Autodesk Inventor part; units mm, degrees
ref_plane "YZ Plane" through (0, 0, 0) normal (1, 0, 0) x (0, 1, 0)
ref_plane "XZ Plane" through (0, 0, 0) normal (0, 1, 0) x (-1, 0, 0)
ref_plane "XY Plane" through (0, 0, 0) normal (0, 0, 1) x (1, 0, 0)
sketch "Sketch1" plane through (0, 0, 0) normal (0, 1, 0) x (-1, 0, 0)
  line L0 (13, -39.6468) -> (13, 41.6738)
  line L1 (13, 41.6738) -> (-0.1234, 53.6991)
  line L2 (-0.1234, 53.6991) -> (-13, 39.6468)
  line L3 (-13, 39.6468) -> (-13, -41.6738)
  line L4 (-13, -41.6738) -> (0.1234, -53.6991)
  line L5 (0.1234, -53.6991) -> (13, -39.6468)
  line L6 (-9.6864, 40.3026) -> (-3.378, 47.187)
  arc A0 (3.6864, 47.4955) -> (-3.378, 47.187) centre (0.3084, 43.8091) ccw
  line L7 (3.6864, 47.4955) -> (9.378, 42.2801)
  arc A1 (11, 38.5937) -> (9.378, 42.2801) centre (6, 38.5937) ccw
  line L8 (11, 38.5937) -> (11, -36.9246)
  arc A2 (9.6864, -40.3026) -> (11, -36.9246) centre (6, -36.9246) ccw
  line L9 (9.6864, -40.3026) -> (3.378, -47.187)
  arc A3 (-3.6864, -47.4955) -> (3.378, -47.187) centre (-0.3084, -43.8091) ccw
  line L10 (-3.6864, -47.4955) -> (-9.378, -42.2801)
  arc A4 (-11, -38.5937) -> (-9.378, -42.2801) centre (-6, -38.5937) ccw
  line L11 (-11, -38.5937) -> (-11, 36.9246)
  arc A5 (-9.6864, 40.3026) -> (-11, 36.9246) centre (-6, 36.9246) ccw
  line L12 (12.8, -39.569) -> (0.111, -53.4166)
  line L13 (0.111, -53.4166) -> (-12.8, -41.5858)
  line L14 (-12.8, -41.5858) -> (-12.8, 39.569)
  line L15 (-12.8, 39.569) -> (-0.111, 53.4166)
  point P0 (0, 0)
  point P1 (0, 0)
extrude "Extrusion1" add sketch "Sketch1" along normal blind 0.4 contours L5 L4 L3 L2 L1 L0 | L6 A0 L7 A1 L8 A2 L9 A3 L10 A4 L11 A5
properties part number "g"
Work out the finished part from the listing and answer in its coordinate system (mm). Give positions to 0.01 mm unless a question says otherwise; leave off trailing zeros. Loops run counter-clockwise (first coordinate to the right, second up) from the corner with the lowest first, then second, coordinate; pieces in that order, holes last. Notation, with made-up numbers: (-28.5, 24.25) -> (-23.5, 24.25) arc R13 cw to (-23.5, 40.25) -> close; hole circle Ø8 at (73.25, 29). An arc over 180 degrees is marked (long way). Use a Markdown table: item, result. Add a question column.
1) Consider line 1 along Z through (x, y) = (3.25, 0.2); line 2 along Z through (x, y) = (-11.5, 0.35); line 3 along X through (y, z) = (0.2, -43.5). Determine where each line is inside the solid, lowest interval first.
2) The part is cut by section C-C, the plane z = 44. Determine the outline of the cut face in (x, y), plus the area to 3 significant figures.
3) The part is cut by section A-A, the plane y = 0.1. Determine the outline of the cut face in (x, z).
4) The part is cut by section B-B, the plane x = 11.5. Determine the outline of the cut face in (y, z), plus the area to 3 significant figures.
Reported:
| question | item | result |
|---|---|---|
| 1 | line 1 | z = -50.61 to 50.29 |
| 1 | line 2 | z = -41.28 to 43.05 |
| 1 | line 3 | x = -9.47 to 11.01 |
| 2 | outline | (-10.46, 0) -> (9.01, 0) -> (9.01, 0.4) -> (-10.46, 0.4) -> close |
| 2 | area | 7.79 mm^2 |
| 3 | outline | (-13, -39.65) -> (-0.12, -53.7) -> (13, -41.67) -> (13, 39.65) -> (0.12, 53.7) -> (-13, 41.67) -> close |
| 4 | outline | (0, -43.05) -> (0.4, -43.05) -> (0.4, 41.28) -> (0, 41.28) -> close |
| 4 | area | 33.7 mm^2 |
